Design review of the part built by this model. Coordinates are the model's own, in mm. A direction names the side the tool comes from. Round coordinates to 2 decimals unless told otherwise and drop trailing zeros. Loops run counter-clockwise (first coordinate to the right, second up) from the corner with the lowest first, then second, coordinate; pieces in that order, holes last. Notation, with made-up numbers: (9, 11.5) - (44, 11.5) arc R25 cw to (44, 27.5) - close; hole circle Ø7 at (36, -23). An arc over 180 degrees is marked (long way). Return JSON: item names as keys, results as strings. Group by question number.
(1) Wall thickness on L1, parallel to Y at x = 2, z = 12; L2, parallel to Z at x = 101, y = -0.5; L3, parallel to Z at x = 57.5, y = -2.75: over which ranges is each line inside the solid? List them lowest first. Write a range as [from, to].
(2) We need section C-C, the plane z = 25. Write out the cut boundary in (x, y), and give its area (3 significant figures).
(3) We need section D-D, the plane z = 12. Write out the cut boundary in (x, y).
(4) We need section B-B, the plane x = -4.5. Write out the cut boundary in (y, z).
(5) Clearance check with flat-ended pins moving along their axes: pin 1 (3 mm diameter, centred on x = -9.5, y = -2, fed in from -Z); pin 2 (2 mm diameter, centred on y = -5, z = 4, fed in from -X). State where each tip first meets the part, or that it passes through.
(6) The part is to be moulded in two halves that separate along X. For faces 1 (the flat face through (-68.232, -1.545, 20.285)), 2 (the flat face through (23, -6.858, 18)), 3 (the flat face through (77.704, -3.381, 24.365)), 4 (the flat face through (72.9, -3.38, 3.92)), say which applies: pulls with the +X half, pulls with the -X half, needs draft (parallel to the pull), parting line crosses it, or undercut.
(7) For faces 5 (the flat face through (23.36, -3.38, 5.3)), 6 (the flat face through (-22.121, -5.355, 13.503)), 7 (the flat face through (14.601, -3.381, 7.543)), 8 (the flat face through (-22.121, -1.545, 13.344)), list the 3-axis set-ups (+Z, -Z, +X, -X, +Y, -Y) from which the entire face can be reached by the end or side of a thin tool; tool diameter is ignored.
(8) We need section A-A, the plane y = -1.75. Write out the cut boundary in (x, z).
from build123d import *

# Parameters (mm, degrees)
F1_DEPTH = 6.858
F4_SIZE2 = 11.3752908615
F4_SIZE  = 3.048
F5_SIZE2 = 3.048
F5_SIZE  = 11.3752908615


with BuildPart() as f1:
    # F0 (on Front) → F1 (new body)
    with BuildSketch(Plane.XZ):
        Polygon((25.9381346405, 7.736035157), (14.33934737, 7.736035157), (20.8550654352, 2.9368868563), align=None)
        Polygon((-53.0272046242, 35.0727677199), (-91.5240803441, 27.1352675399), (-57.573735714, 7.736035157), (14.33934737, 7.736035157), (25.9381346405, 7.736035157), (121.1881346405, 0), (124.3759196559, 6.8946417749), (118.7927769162, 20.2559313961), (35.4490326759, 28.5903061262), (27.808678696, 32.9560056193), align=None)
    extrude(amount=F1_DEPTH)

    # F4
    f4_edges = [f1.edges().sort_by_distance(p)[0] for p in [
        (-74.548908, -6.858, 17.435651),
        (-21.617194, -6.858, 7.736035),
    ]]
    chamfer(f4_edges, length=F4_SIZE, length2=F4_SIZE2)

    # F5
    f5_edges = [f1.edges().sort_by_distance(p)[0] for p in [
        (-74.548908, 0, 17.435651),
        (-21.617194, 0, 7.736035),
    ]]
    f5_side = f1.faces().sort_by_distance((17.333868, 0, 18.236696))[0]
    chamfer(f5_edges, length=F5_SIZE, length2=F5_SIZE2, reference=f5_side)


solid = f1.part
Solutions:
{
 "1": {"L1": "[-4.95, -1.91]", "L2": "[1.64, 22.04]", "L3": "[5.17, 26.39]"},
 "2": {"outline": "(-87.79, -3.81) - (-64.86, -6.86) - (71.35, -6.86) - (71.35, 0) - (-64.86, 0) - (-87.79, -3.05) - close", "area": "1,020 mm^2"},
 "3": {"outline": "(-65.04, -3.81) - (-56.44, -4.95) - (8.55, -4.95) - (8.55, -6.86) - (122.24, -6.86) - (122.24, 0) - (8.55, 0) - (8.55, -1.91) - (-56.44, -1.91) - (-65.04, -3.05) - close"},
 "4": {"outline": "(-6.86, 19.11) - (-3.81, 7.74) - (-3.05, 7.74) - (0, 19.11) - (0, 33.8) - (-6.86, 33.8) - close"},
 "5": {"pin 1": "z = 7.74", "pin 2": "x = 18.05"},
 "6": {"face 1": "pulls with the -X half", "face 2": "needs draft", "face 3": "pulls with the +X half", "face 4": "undercut"},
 "7": {"face 5": "-Z, +Y, -Y", "face 6": "-Z, -X, -Y", "face 7": "-Z, -X", "face 8": "-Z, -X, +Y"},
 "8": {"outline": "(-84.35, 28.61) - (-56.29, 12.58) - (7.76, 12.58) - (20.86, 2.94) - (25.94, 7.74) - (121.19, 0) - (124.38, 6.89) - (118.79, 20.26) - (35.45, 28.59) - (27.81, 32.96) - (-53.03, 35.07) - close"}
}
